Check sheet for the modelled part. Datum: model origin and axes. Units: mm. A direction names the side the tool comes from. Give positions to 0.01 mm unless a question says otherwise; leave off trailing zeros. Order: outer loops, then holes, each group sorted by start corner. A loop starts at its lowest first (then second) coordinate and runs counter-clockwise, first axis right, second up. Notation, with made-up numbers: M 60,67.5 L 109,67.5 A10 cw 109,83.5 Z; hole C 56,35 d2. An arc over 180 degrees is marked long. Answer in a Markdown table with one row per item. Add a question column.
from build123d import *

# Parameters (mm, degrees)
F0_W     = 20
F0_H     = 20
F1_DEPTH = 4
F3_DEPTH = 3.1
F4_W     = 20
F4_H     = 20
F5_DEPTH = 4
F6_R     = 2.25
F7_DEPTH = 25


with BuildPart() as f1:
    # F0 (on Top) → F1 (new body)
    with BuildSketch(Plane.XY):
        with Locations((10, -10)):
            Rectangle(F0_W, F0_H)
    extrude(amount=F1_DEPTH)

    # F2 (on face) → F3 (join)
    with BuildSketch(Plane.XY.offset(4)):
        Polygon((20, 0), (0, 0), (7.101437, -7.101437), (11.060948, -6.040489), (12.510229, -7.489771), align=None)
        Polygon((12.898563, -12.898563), (20, -20), (20, 0), (12.510229, -7.489771), (13.959511, -8.939052), align=None)
        Polygon((0, 0), (0, -20), (7.489771, -12.510229), (6.040489, -11.060948), (7.101437, -7.101437), align=None)
        Polygon((7.489771, -12.510229), (0, -20), (20, -20), (12.898563, -12.898563), (8.939052, -13.959511), align=None)
    extrude(amount=F3_DEPTH)

    # F4 (on face) → F5 (join)
    with BuildSketch(Plane.XY.offset(7.1)):
        with Locations((10, -10)):
            Rectangle(F4_W, F4_H)
    extrude(amount=F5_DEPTH)

    # F6 (on face) → F7 (cut)
    with BuildSketch(Plane.XY.offset(11.1)):
        with Locations((10, -10)):
            Circle(F6_R)
    extrude(amount=-F7_DEPTH, mode=Mode.SUBTRACT)


solid = f1.part
Q1. Tool access check on faces 1 (the flat face through (9.05, -6.58, 5.53)), 2 (the flat face through (0, -10, 5)). Record the directions out of +Z, -Z, +X, -X, +Y, -Y that give a thin tool (end or side, any length) a straight path to the whole face; none if there is none.
Q2. Go/stop test with a flat-tipped pin: pin 1 (1.5 mm diameter, centred on x = 12, y = -5, fed in from -Z). Record where the tip stops, or that it passes through.
Q3. Cross-section at A-A (x = 10). Record the boundary of the cut face in (y, z).
Q4. Cross-section at C-C (y = -10). Record the boundary of the cut face in (x, z), and give its area (3 significant figures).
Q5. Thickness scan on probe 1 along Y at (x, z) = (10, 8.65); probe 2 along Z at (x, y) = (11.5, -7.75); probe 3 along X at (y, z) = (-8, 10). Record the ranges inside material, lowest first.
Q6. Cross-section at D-D (x = 6.5). Record the boundary of the cut face in (y, z), and give its area (3 significant figures).
Q7. Draft check along Z on faces 3 (the flat face through (20, -10, 5)), 4 (the flat face through (9.9, -7.6, 0)), 5 (the flat face through (6.564, -9.109, 5.528)). Enter one of: pulls with the +Z half, pulls with the -Z half, needs draft (parallel to the pull), parting line crosses it, or undercut.
Q8. Cross-section at B-B (z = 10). Record the boundary of the cut face in (x, y), and give its area (3 significant figures).
Values follow:
| question | item | result |
|---|---|---|
| 1 | face 1 | none |
| 1 | face 2 | +Z, -Z, -X, +Y, -Y |
| 2 | pin 1 | z = 0 |
| 3 | outline | M -20,0 L -12.25,0 L -12.25,4 L -13.68,4 L -13.68,7.1 L -12.25,7.1 L -12.25,11.1 L -20,11.1 Z; M -7.75,0 L 0,0 L 0,11.1 L -7.75,11.1 L -7.75,7.1 L -6.32,7.1 L -6.32,4 L -7.75,4 Z |
| 4 | outline | M 0,0 L 7.75,0 L 7.75,4 L 6.32,4 L 6.32,7.1 L 7.75,7.1 L 7.75,11.1 L 0,11.1 Z; M 12.25,0 L 20,0 L 20,11.1 L 12.25,11.1 L 12.25,7.1 L 13.68,7.1 L 13.68,4 L 12.25,4 Z |
| 4 | area | 163 mm² |
| 5 | probe 1 | -20 to -12.25, -7.75 to 0 |
| 5 | probe 2 | 0 to 4, 7.1 to 11.1 |
| 5 | probe 3 | 0 to 8.97, 11.03 to 20 |
| 6 | outline | M -20,0 L 0,0 L 0,11.1 L -20,11.1 Z; hole M -11.52,4 L -9.35,4 L -9.35,7.1 L -11.52,7.1 Z |
| 6 | area | 215 mm² |
| 7 | face 3 | needs draft |
| 7 | face 4 | pulls with the -Z half |
| 7 | face 5 | undercut |
| 8 | outline | M 0,-20 L 20,-20 L 20,0 L 0,0 Z; hole C 10,-10 d4.5 |
| 8 | area | 384 mm² |
